from build123d import *

# Parameters (mm, degrees)
EXTRUDE_1_DEPTH     = 1
CUT_EXTRUDE_1_DEPTH = 10
FILLET_1_R          = 2
FILLET_2_R          = 2


with BuildPart() as part:
    # 草图1 → 凸台-拉伸1 (new body)
    with BuildSketch(Plane(origin=(-61.5, 0, 0), x_dir=(0, -1, 0), z_dir=(-1, 0, 0))):
        with BuildLine():
            Line((145.112990447, 800.603209432), (176.378367534, 797.698696456))
            ThreePointArc((176.378367534, 797.698696456), (177.840703349, 798.15115608), (178.554793652, 799.505120921))
            Line((178.554793652, 799.505120921), (187.157332086, 892.106397006))
            Line((187.157332086, 892.106397006), (-47.830852387, 913.936494537))
            Line((-47.830852387, 913.936494537), (-56.433390821, 821.335218452))
            ThreePointArc((-56.433390821, 821.335218452), (-55.980931196, 819.872882636), (-54.626966355, 819.158792334))
            Line((-54.626966355, 819.158792334), (-23.361589268, 816.254279357))
            ThreePointArc((-23.361589268, 816.254279357), (-17.376417442, 821.221946637), (-12.408750162, 815.236774811))
            Line((-12.408750162, 815.236774811), (20.848052217, 812.147261008))
            Line((20.848052217, 812.147261008), (25.288072054, 859.941468019))
            Line((25.288072054, 859.941468019), (26.482927229, 859.830467523))
            Line((26.482927229, 859.830467523), (22.042907393, 812.036260512))
            Line((22.042907393, 812.036260512), (55.399281036, 808.937496668))
            ThreePointArc((55.399281036, 808.937496668), (61.384452862, 813.905163948), (66.352120143, 807.919992122))
            Line((66.352120143, 807.919992122), (99.708493786, 804.821228277))
            Line((99.708493786, 804.821228277), (104.148513623, 852.615435289))
            Line((104.148513623, 852.615435289), (105.343368798, 852.504434793))
            Line((105.343368798, 852.504434793), (100.903348961, 804.710227781))
            Line((100.903348961, 804.710227781), (134.16015134, 801.620713978))
            ThreePointArc((134.16015134, 801.620713978), (140.145323166, 806.588381259), (145.112990447, 800.603209432))
        make_face()
    extrude(amount=-EXTRUDE_1_DEPTH)

    # 草图2 → 切除-拉伸1 (cut)
    with BuildSketch(Plane(origin=(-60.5, 0, 0), x_dir=(0, 0, -1), z_dir=(1, 0, 0))):
        Polygon((-804.821228277, -99.708493786), (-899.413929654, -108.496033046), (-892.106397006, -187.157332086), (-797.513695629, -178.369792826), align=None)
    extrude(amount=-CUT_EXTRUDE_1_DEPTH, mode=Mode.SUBTRACT)

    # 圆角1
    fillet_1_edges = [part.edges().sort_by_distance(p)[0] for p in [
        (-61, -108.496033046, 899.413929654),
    ]]
    fillet(fillet_1_edges, radius=FILLET_1_R)

    # 圆角2
    fillet_2_edges = [part.edges().sort_by_distance(p)[0] for p in [
        (-61, -99.708493786, 804.821228277),
    ]]
    fillet(fillet_2_edges, radius=FILLET_2_R)


solid = part.part
The model under review builds one solid part; all positions refer to its coordinate system, in mm. A direction names the side the tool comes from. Give positions to 0.01 mm unless a question says otherwise; leave off trailing zeros. Write each loop counter-clockwise with the first axis right and the second up, starting at its lowest first coordinate (ties: lowest second). Pieces come first, ordered by that corner, then holes.
1. Add section C-C, the plane y = 10. Write out the cut boundary in (x, z).
2. Add section B-B, the plane z = 830. Write out the cut boundary in (x, y).
3. Draft analysis for pull direction Y (two halves, no side actions). For faces 3 (the flat face through (-61.01, -38.49, 810.51)), 4 (the flat face through (-61.007, -24.294, 836.268)), 5 (the flat face through (-61.007, -30.417, 906.667)), state which applies: +Y half, -Y half, draft (parallel to the pull), parting line (faces both ways), or undercut.
4. Tool access review of faces 1 (the flat face through (-61.5, -25, 860)), 2 (the flat face through (-61.007, -23.037, 835.71)): name each direction out of +Z, -Z, +X, -X, +Y, -Y from which nothing blocks a thin tool from reaching the whole face with its end or side.
5. Add section A-A, the plane x = -60.8. Write out the cut boundary in (y, z), plus the area to 3 significant figures.
6. Wall thickness on L1, parallel to Y at x = -61.15, z = 848; L2, parallel to Y at x = -60.85, z = 858; L3, parallel to Z at x = -60.85, y = -13: over which ranges is each line inside the solid? List them lowest first.
7. Add section D-D, the plane z = 866.5. Write out the cut boundary in (x, y).
Worked answers:
1. outline: (-61.5, 815.01) - (-60.5, 815.01) - (-60.5, 910.42) - (-61.5, 910.42) - close
2. outline: (-61.5, -102.05) - (-60.5, -102.05) - (-60.5, -23.71) - (-61.5, -23.71) - close; (-61.5, -22.51) - (-60.5, -22.51) - (-60.5, 55.63) - (-61.5, 55.63) - close
3. face 3: +Y half
3. face 4: undercut
3. face 5: -Y half
4. face 1: +Z, -Z, -X, +Y, -Y
4. face 2: +X, -X
5. outline: (-108.31, 897.42) - (-99.89, 806.81) arc R2 ccw to (-97.72, 805.01) - (-66.35, 807.92) arc R5.5 cw to (-55.4, 808.94) - (-22.04, 812.04) - (-26.48, 859.83) - (-25.29, 859.94) - (-20.85, 812.15) - (12.41, 815.24) arc R5.5 cw to (23.36, 816.25) - (54.63, 819.16) arc R2 ccw to (56.43, 821.34) - (47.83, 913.94) - (-106.5, 899.6) arc R2 ccw to start
5. area: 14,800 mm2
6. L1: y = -103.72 to -25.38, -24.18 to 53.96
6. L2: y = -104.65 to -26.31, -25.11 to 53.03
6. L3: z = 812.88 to 908.29
7. outline: (-61.5, -105.44) - (-60.5, -105.44) - (-60.5, 52.24) - (-61.5, 52.24) - close
